from build123d import *

# Parameters (mm, degrees)
SKETCH_1_R      = 2.1
EXTRUDE_1_DEPTH = 8.5
FILLET_1_R      = 0.3


with BuildPart() as part:
    # 草图1 → 凸台-拉伸1 (new body)
    with BuildSketch(Plane(origin=(0, 0, 0), x_dir=(1, 0, 0), z_dir=(0, 1, 0))):
        with BuildLine():
            ThreePointArc((-3.125, 5.412658774), (-1.246843801, 4.653284414), (0, 6.25))
            ThreePointArc((0, 6.25), (1.246843801, 4.653284414), (3.125, 5.412658774))
            ThreePointArc((3.125, 5.412658774), (3.406440613, 3.406440613), (5.412658774, 3.125))
            ThreePointArc((5.412658774, 3.125), (4.653284414, 1.246843801), (6.25, 0))
            ThreePointArc((6.25, 0), (4.653284414, -1.246843801), (5.412658774, -3.125))
            ThreePointArc((5.412658774, -3.125), (3.406440613, -3.406440613), (3.125, -5.412658774))
            ThreePointArc((3.125, -5.412658774), (1.246843801, -4.653284414), (0, -6.25))
            ThreePointArc((0, -6.25), (-1.246843801, -4.653284414), (-3.125, -5.412658774))
            ThreePointArc((-3.125, -5.412658774), (-3.406440613, -3.406440613), (-5.412658774, -3.125))
            ThreePointArc((-5.412658774, -3.125), (-4.653284414, -1.246843801), (-6.25, 0))
            ThreePointArc((-6.25, 0), (-4.653284414, 1.246843801), (-5.412658774, 3.125))
            ThreePointArc((-5.412658774, 3.125), (-3.406440613, 3.406440613), (-3.125, 5.412658774))
        make_face()
        Circle(SKETCH_1_R, mode=Mode.SUBTRACT)
    extrude(amount=EXTRUDE_1_DEPTH)

    # 圆角1
    fillet_1_edges = [part.edges().sort_by_distance(p)[0] for p in [
        (-3.125, 4.25, -5.412658774),
        (0, 4.25, -6.25),
        (3.125, 4.25, -5.412658774),
        (5.412658774, 4.25, -3.125),
        (6.25, 4.25, 0),
        (5.412658774, 4.25, 3.125),
        (3.125, 4.25, 5.412658774),
        (0, 4.25, 6.25),
        (-3.125, 4.25, 5.412658774),
        (-5.412658774, 4.25, 3.125),
        (-6.25, 4.25, 0),
        (-5.412658774, 4.25, -3.125),
    ]]
    fillet(fillet_1_edges, radius=FILLET_1_R)


solid = part.part
Work out the finished part from the listing and answer in its coordinate system (mm). Round coordinates to 2 decimals unless told otherwise and drop trailing zeros. Write each loop counter-clockwise with the first axis right and the second up, starting at its lowest first coordinate (ties: lowest second). Pieces come first, ordered by that corner, then holes. Notation, with made-up numbers: (-24.75, -5.75) - (-8.75, -5.75) arc R13 cw to (-8.75, 8.25) - close; hole circle Ø10 at (-16, -34). An arc over 180 degrees is marked (long way). Answer in a Markdown table with one row per item. Add a question column.
1. Given pin 1 (1.5 mm diameter, centred on y = 6.5, z = 3.5, fed in from +X); pin 2 (2 mm diameter, centred on x = 4.5, y = 6.5, fed in from +Z), each flat-ended and moving along its own axis, determine where each tip first touches the part or whether it passes through.
2. Find the intervals of material crossed by line 1 along Z through (x, y) = (0, 3.75); line 2 along X through (y, z) = (4.5, 1.5), in increasing order. Write a range as from..to.
3. A cutting plane is placed at B-B, the plane x = 1.75. Determine the outline of the cut face in (y, z), and give its area (3 significant figures).
4. The mould has two halves that part along Z. Classify faces 1 (the cylindrical face through (3.394, 4.19, -3.419)), 2 (the cylindrical face through (2.003, 4.19, -0.631)), 3 (the cylindrical face through (3.419, 4.19, 3.394)): +Z half, -Z half, draft (parallel to the pull), parting line (faces both ways), or undercut.
5. A cutting plane is placed at A-A, the plane x = -0.75. Determine the outline of the cut face in (y, z).
Worked out:
| question | item | result |
|---|---|---|
| 1 | pin 1 | x = 4.8 |
| 1 | pin 2 | z = 3.32 |
| 2 | line 1 | -5.53..-2.1, 2.1..5.53 |
| 2 | line 2 | -4.61..-1.47, 1.47..4.61 |
| 3 | outline | (0, -4.6) - (8.5, -4.6) - (8.5, -1.16) - (0, -1.16) - close; (0, 1.16) - (8.5, 1.16) - (8.5, 4.6) - (0, 4.6) - close |
| 3 | area | 58.4 mm^2 |
| 4 | face 1 | -Z half |
| 4 | face 2 | undercut |
| 4 | face 3 | +Z half |
| 5 | outline | (0, -4.88) - (8.5, -4.88) - (8.5, -1.96) - (0, -1.96) - close; (0, 1.96) - (8.5, 1.96) - (8.5, 4.88) - (0, 4.88) - close |
